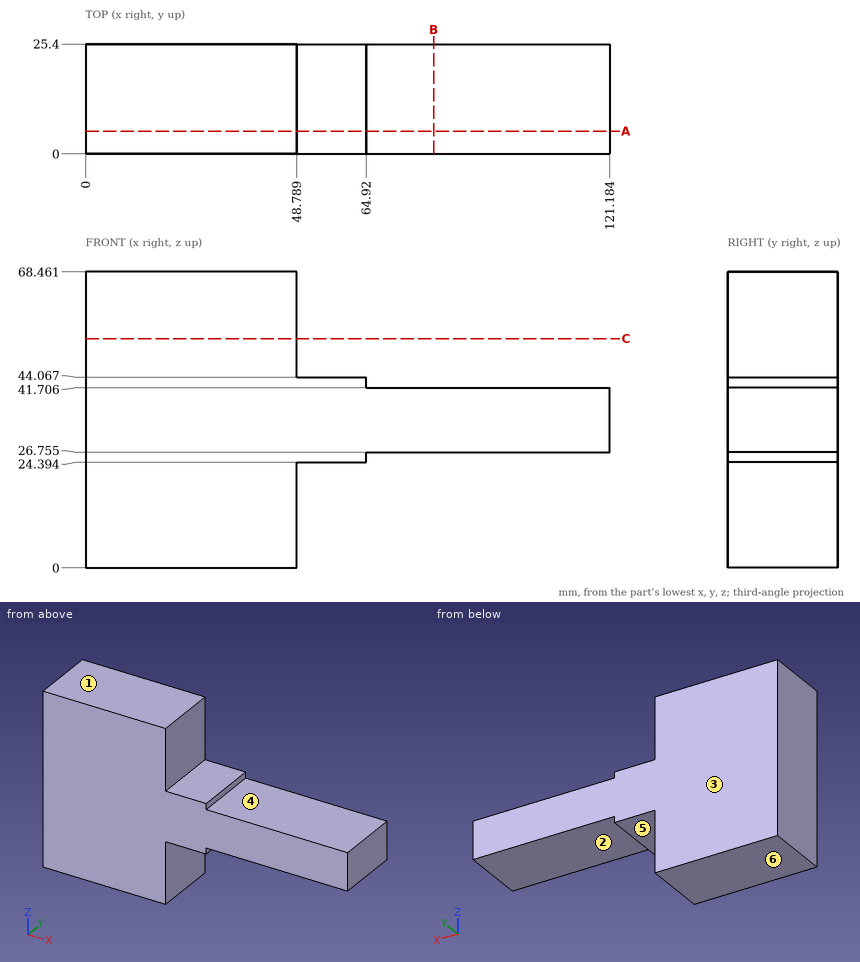
Source: three-view drawing plus pictorial views. Frame: mm from the lowest corner of the part. A direction names the side the tool comes from. Give positions to 0.01 mm unless a question says otherwise; leave off trailing zeros. Order: outer loops, then holes, each group sorted by start corner. A loop starts at its lowest first (then second) coordinate and runs counter-clockwise, first axis right, second up. Notation, with made-up numbers: (76.5, -4) - (132.5, -4) arc R18 cw to (132.5, 19) - close; hole circle Ø11 at (-8.5, 69). An arc over 180 degrees is marked (long way). Put each result on its own line as item: value.
Item 1: Contact query for flat-ended pins moving along their axis: pin 1 (12 mm diameter, centred on y = 12, z = 61.5, fed in from +X); pin 2 (2 mm diameter, centred on x = 45, y = 15, fed in from -Z); pin 3 (5 mm diameter, centred on x = 59, y = 12.5, fed in from +Z); pin 4 (0.7 mm diameter, centred on y = 7, z = 43.5, fed in from +X). Output: stop coordinate, or through.
Found:
pin 1: stops at x = 48.79
pin 2: stops at z = 0
pin 3: stops at z = 44.07
pin 4: stops at x = 64.92
Item 2: Access query for the marked faces 4, 5 and 6. Directions: +Z, -Z, +X, -X, +Y, -Y. A direction counts if a zero-diameter tool reaches every point of the face in a straight line with its end or side. Return the directions, or none.
Found:
face 4: +Z, +X, +Y, -Y
face 5: -Z, +X, +Y, -Y
face 6: -Z, +X, -X, +Y, -Y
Item 3: Draft query along Z for the marked faces 1, 2 and 3. Return one class per face: +Z half, -Z half, draft (parallel to the pull), parting line (faces both ways), or undercut.
Found:
face 1: +Z half
face 2: -Z half
face 3: draft
Item 4: Section query A-A, the plane y = 5.25. Return loops of the section in (x, z) (1 decimal), then the cut area to 3 significant figures.
Found:
outline: (0, 0) - (48.8, 0) - (48.8, 24.4) - (64.9, 24.4) - (64.9, 26.8) - (121.2, 26.8) - (121.2, 41.7) - (64.9, 41.7) - (64.9, 44.1) - (48.8, 44.1) - (48.8, 68.5) - (0, 68.5) - close
area: 4,500 mm^2
Item 5: Section query B-B, the plane x = 80.5. Return loops of the section in (y, z) (1 decimal).
Found:
outline: (0, 26.8) - (25.4, 26.8) - (25.4, 41.7) - (0, 41.7) - close
Item 6: Section query C-C, the plane z = 53. Return loops of the section in (x, y).
Found:
outline: (0, 0) - (48.79, 0) - (48.79, 25.4) - (0, 25.4) - close
Item 7: Ray query, L1, parallel to Z at x = 54, y = 7.75 (1 decimal); L2, parallel to Z at x = 115, y = 9.5 (1 decimal); L3, parallel to X at y = 20.25, z = 24.5. Return the intervals inside material, ascending. Write a range as from..to.
Found:
L1: z = 24.4..44.1
L2: z = 26.8..41.7
L3: x = 0..64.92
